Geometry check sheet. Reference: the model listing, model coordinates, mm. Round coordinates to 2 decimals unless told otherwise and drop trailing zeros. Order: outer loops, then holes, each group sorted by start corner. A loop starts at its lowest first (then second) coordinate and runs counter-clockwise, first axis right, second up.
(1) Thickness scan on L1, parallel to Z at x = -9, y = 3.5; L2, parallel to X at y = -1.5, z = 3; L3, parallel to X at y = 0, z = 6. Record the ranges inside material, lowest first.
(2) Cross-section at A-A on x = 0. Enter the section's corners in (y, z).
(3) Gauge pin test, flat ends, axial feed: P1, Ø6, axis at y = -2, z = 3.5, coming from the +X side; P2, Ø8, axis at y = 1, z = -5.5, coming from the +X side; P3, Ø3, axis at y = -1, z = 12.5, coming from the -X side. Record the tip position at first contact, or that the pin passes through.
(4) Cross-section at C-C on y = -3. Enter the section's corners in (x, z), and give its area (3 significant figures).
(5) Cross-section at B-B on z = 0. Enter the section's corners in (x, y), and give its area (3 significant figures).
(6) Cross-section at D-D on y = 2.25. Enter the section's corners in (x, z), and give its area (3 significant figures).
from build123d import *

# Parameters (mm, degrees)
SZKIC1_R                    = 16
DODANIE_WYCI_GNI_CIE1_DEPTH = 7.5
ZAOKR_GLENIE1_R             = 0.2


with BuildPart() as part:
    # Szkic1 → Dodanie-wyciągnięcie1 (new, symmetric)
    with BuildSketch(Plane(origin=(0, 0, 0), x_dir=(1, 0, 0), z_dir=(0, 1, 0))):
        with Locations(Location((0, 0, 0), (0, 0, 270))):
            Circle(SZKIC1_R)
    extrude(amount=DODANIE_WYCI_GNI_CIE1_DEPTH, both=True)

    # Szkic3 → Wycięcie-obrót1 (revolve, cut)
    with BuildSketch(Plane.XY):
        with BuildLine():
            Line((0, -14.26), (0, 14.26))
            ThreePointArc((0, 14.26), (14.26, 0), (0, -14.26))
        make_face()
    revolve(axis=Axis((0, -14.26, 0), (0, 1, 0)), mode=Mode.SUBTRACT)

    # Zaokrąglenie1
    zaokr_glenie1_edges = [part.edges().sort_by_distance(p)[0] for p in [
        (0, -7.5, -16),
        (0, 7.5, -16),
    ]]
    fillet(zaokr_glenie1_edges, radius=ZAOKR_GLENIE1_R)


solid = part.part
Found:
1. L1: z = -13.23 to -10.49, 10.49 to 13.23
1. L2: x = -15.72 to -13.86, 13.86 to 15.72
1. L3: x = -14.83 to -12.94, 12.94 to 14.83
2. outline: (-7.5, -15.8) arc R0.2 ccw to (-7.3, -16) - (7.3, -16) arc R0.2 ccw to (7.5, -15.8) - (7.5, -12.13) arc R14.26 cw to (-7.5, -12.13) - close; (-7.5, 12.13) arc R14.26 cw to (7.5, 12.13) - (7.5, 15.8) arc R0.2 ccw to (7.3, 16) - (-7.3, 16) arc R0.2 ccw to (-7.5, 15.8) - close
3. P1: stops at x = 15.99
3. P2: stops at x = 15.93
3. P3: stops at x = -11.62
4. outline: circle Ø32 at (0, 0); hole circle Ø27.88 at (0, 0)
4. area: 194 mm2
5. outline: (-16, -7.3) arc R0.2 ccw to (-15.8, -7.5) - (-12.13, -7.5) arc R14.26 cw to (-12.13, 7.5) - (-15.8, 7.5) arc R0.2 ccw to (-16, 7.3) - close; (12.13, -7.5) - (15.8, -7.5) arc R0.2 ccw to (16, -7.3) - (16, 7.3) arc R0.2 ccw to (15.8, 7.5) - (12.13, 7.5) arc R14.26 cw to start
5. area: 72.8 mm2
6. outline: circle Ø32 at (0, 0); hole circle Ø28.16 at (0, 0)
6. area: 181 mm2
